CAD build for the part. Positions are in the model's coordinates, mm. Face numbers are marked on the shaded views. A direction names the side the tool comes from. Coordinates: 2 decimals unless noted, no trailing zeros. Write each loop counter-clockwise with the first axis right and the second up, starting at its lowest first coordinate (ties: lowest second). Pieces come first, ordered by that corner, then holes. Notation, with made-up numbers: (47, -5.5) - (78, -5.5) arc R23 ccw to (78, 17.5) - close; hole circle Ø7 at (48, 79.5). An arc over 180 degrees is marked (long way). One line per question, with ' | ' between items. Start each with the question number.
1. Band-saw the part on D-D, the plane y = 6. Write the cut outline in (x, z).
2. Which spindle directions (+Z, -Z, +X, -X, +Y, -Y) get a long thin tool onto all of the face, cutting with end or side? Do the marked faces 1, 2, 3 and 4. Say none if no direction does.
3. Band-saw the part on C-C, the plane x = -11. Write the cut outline in (y, z), then the cut area to 3 significant figures.
4. Band-saw the part on A-A, the plane y = -24. Write the cut outline in (x, z).
5. Band-saw the part on B-B, the plane x = -42.5. Write the cut outline in (y, z).
6. Flat gauge pins, fed straight in: P1, Ø12.5, axis at x = -36, z = 45.5, coming from the +Y side; P2, Ø12, axis at y = -32, z = 31, coming from the +X side; P3, Ø1.5, axis at y = -23.5, z = 8.5, coming from the +X side; P4, Ø17, axis at y = -5.5, z = 54, coming from the -X side. Where does each tip first touch, or does it go through?
7. Probe line 1 (X direction, y = -26, z = 34); line 2 (X direction, y = -23, z = 52); line 3 (Y direction, x = -19, z = 20.5). List the from-to ranges inside material, lowest first.
8. Two-plate mould, pull along X, no slides. Class the marked faces 5, 6 and 7: +X half, -X half, draft (parallel to the pull), parting line (faces both ways), or undercut.
from build123d import *

# Parameters (mm, degrees)
F1_DEPTH     = 76.2
F2_DEPTH     = 15.24
F3_R         = 12.8774151417
F4_R         = 20.6186868219
F5_T1_DEPTH  = 101.180790156
F6_R         = 2.2113922374
F7_T1_DEPTH  = 154.3936506005
F8_T1_DEPTH  = 132.0243451665
F9_T1_DEPTH  = 76.2
F10_T1_DEPTH = 168.1440052245
F11_R        = 2.3364132001
F12_T        = -5.334


# Not quite as in the source:
# - a fillet or chamfer that OpenCascade refuses, or shapes differently, is made with other operations: its cross-section is extruded or revolved along the edge and cut away or added


with BuildPart() as f1:
    # F0 (on Top) → F1 (new body)
    with BuildSketch(Plane.XY):
        Polygon((-23.9872187376, -31.7199416459), (-47.0275729895, 62.9664510489), (-55.8593086898, 62.9664510489), (-55.8593086898, -44.0704375505), (-69.4310441613, -52.1240867674), (7.9028792679, -52.1240867674), (-21.2087563334, -41.9485626592), (8.002824487, -34.8404117285), (3.777547454, -17.4762585554), (-1.7201294546, -18.8140265274), (0, -25.8830520834), align=None)
    extrude(amount=F1_DEPTH)

    # F2 (cut): a face of the model
    f2_faces = [f1.faces().sort_by_distance(p)[0] for p in [
        (-55.8593086898, 9.4480067492, 38.1),
    ]]
    extrude(f2_faces, amount=-F2_DEPTH, mode=Mode.SUBTRACT)

    # F3
    f3_edges = [f1.edges().sort_by_distance(p)[0] for p in [
        (-40.619309, -44.070438, 38.1),
    ]]
    fillet(f3_edges, radius=F3_R)

    # F4
    f4_edges = [f1.edges().sort_by_distance(p)[0] for p in [
        (-55.859309, -44.070438, 38.1),
    ]]
    fillet(f4_edges, radius=F4_R)

    # F5: fillet of radius 1.3707998783 on 1 edges, made by hand

    # F5_s2 → F5_t1 (cut)
    with BuildSketch(Plane.XY.offset(-12.490395078)):
        with BuildLine():
            ThreePointArc((-65.1344391621, -49.5744239362), (-65.7568311931, -51.1159900142), (-64.4348861301, -52.1240867674))
            Line((-64.4348861301, -52.1240867674), (-69.4310441613, -52.1240867674))
            Line((-69.4310441613, -52.1240867674), (-65.1344391621, -49.5744239362))
        make_face()
    extrude(amount=F5_T1_DEPTH, mode=Mode.SUBTRACT)

    # F6
    f6_edges = [f1.edges().sort_by_distance(p)[0] for p in [
        (-21.208756, -41.948563, 38.1),
    ]]
    fillet(f6_edges, radius=F6_R)

    # F7: fillet of radius 2.6543994462 on 1 edges, made by hand

    # F7_s2 → F7_t1 (cut)
    with BuildSketch(Plane.XY.offset(-39.0968253003)):
        with BuildLine():
            ThreePointArc((-6.8600078332, -46.9639468268), (-5.1188800269, -49.913872102), (-7.7358508522, -52.1240867674))
            Line((-7.7358508522, -52.1240867674), (7.9028792679, -52.1240867674))
            Line((7.9028792679, -52.1240867674), (-6.8600078332, -46.9639468268))
        make_face()
    extrude(amount=F7_T1_DEPTH, mode=Mode.SUBTRACT)

    # F8: fillet of radius 1.3388584964 on 1 edges, made by hand

    # F8_s2 → F8_t1 (cut)
    with BuildSketch(Plane.XY.offset(-27.9121725832)):
        with BuildLine():
            ThreePointArc((-40.6193086898, 25.466247787), (-39.4398601206, 26.7955824133), (-37.979551683, 25.78279974))
            Line((-37.979551683, 25.78279974), (-40.6193086898, 36.6311168203))
            Line((-40.6193086898, 36.6311168203), (-40.6193086898, 25.466247787))
        make_face()
    extrude(amount=F8_T1_DEPTH, mode=Mode.SUBTRACT)

    # F9: fillet of radius 10.4245741623 on 2 edges, made by hand

    # F9_s2 → F9_t1 (join)
    with BuildSketch(Plane.XY):
        with BuildLine():
            ThreePointArc((-26.4519447103, -21.5909302259), (-21.7424015031, -28.031321364), (-13.8582073177, -29.2552156732))
            Line((-13.8582073177, -29.2552156732), (-23.9872187376, -31.7199416459))
            Line((-23.9872187376, -31.7199416459), (-26.4519447103, -21.5909302259))
        make_face()
        with BuildLine():
            ThreePointArc((-9.6557422738, -28.2326159037), (-4.1483336949, -24.8205098096), (-1.7201294546, -18.8140265274))
            Line((-1.7201294546, -18.8140265274), (0, -25.8830520834))
            Line((0, -25.8830520834), (-9.6557422738, -28.2326159037))
        make_face()
    extrude(amount=F9_T1_DEPTH)

    # F10: fillet of radius 18.3963073453 on 1 edges, made by hand

    # F10_s2 → F10_t1 (cut)
    with BuildSketch(Plane.XY.offset(-45.9720026122)):
        with BuildLine():
            ThreePointArc((3.777547454, -17.4762585554), (1.3625814789, -31.1006820929), (-9.8646080702, -39.1881534047))
            Line((-9.8646080702, -39.1881534047), (8.002824487, -34.8404117285))
            Line((8.002824487, -34.8404117285), (3.777547454, -17.4762585554))
        make_face()
    extrude(amount=F10_T1_DEPTH, mode=Mode.SUBTRACT)

    # F11
    f11_edges = [f1.edges().sort_by_distance(p)[0] for p in [
        (3.777547, -17.476259, 38.1),
    ]]
    fillet(f11_edges, radius=F11_R)

    # F12
    f12_openings = [f1.faces().sort_by_distance(p)[0] for p in [
        (-29.256427, -29.797459, 76.2),
        (-29.256427, -29.797459, 0),
    ]]
    offset(amount=F12_T, openings=f12_openings)


solid = f1.part
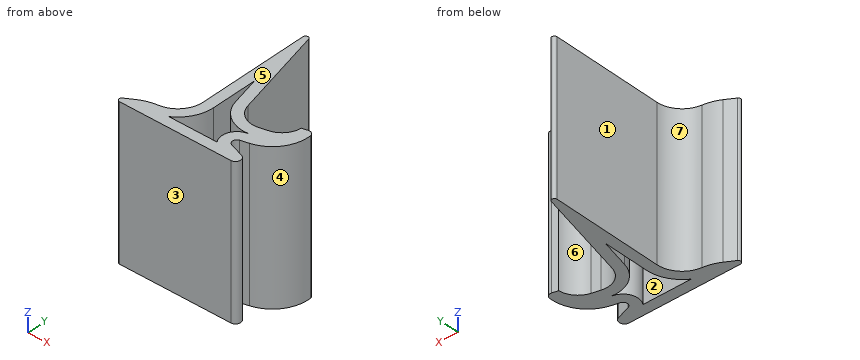
Filled in:
1) outline: (-40.62, 0) - (-33.17, 0) - (-33.17, 76.2) - (-40.62, 76.2) - close
2) face 1: +Z, -Z, -X, +Y | face 2: +Z, -Z | face 3: +Z, -Z, +X, -X, -Y | face 4: +Z, -Z, +X
3) outline: (-52.12, 0) - (-45.52, 0) - (-45.52, 76.2) - (-52.12, 76.2) - close; (-39.46, 0) - (-28.56, 0) - (-28.56, 76.2) - (-39.46, 76.2) - close | area: 1,330 mm²
4) outline: (-40.62, 0) - (-35.29, 0) - (-35.29, 76.2) - (-40.62, 76.2) - close; (-31.31, 0) - (-25.54, 0) - (-25.54, 76.2) - (-31.31, 76.2) - close; (-3.52, 0) - (3.98, 0) - (3.98, 76.2) - (-3.52, 76.2) - close
5) outline: (-52.12, 0) - (-46.79, 0) - (-46.79, 76.2) - (-52.12, 76.2) - close; (-45.71, 0) - (-37.89, 0) - (-37.89, 76.2) - (-45.71, 76.2) - close
6) P1: stops at y = 26.81 | P2: stops at x = 3.58 | P3: stops at x = 4.13 | P4: stops at x = -40.62
7) line 1: x = -40.62 to -35.29, -30.5 to -24.16, -5.31 to 3.58 | line 2: x = -40.62 to -35.29, -31.6 to -26, -2.92 to 4.1 | line 3: y = -52.12 to -37.25, -34.66 to -29.2
8) face 5: draft | face 6: undercut | face 7: -X half
